Study the drawing (mm; zero at the part's minimum x, y, z) and answer. Coordinates: 2 decimals unless noted, no trailing zeros. Order: outer loops, then holes, each group sorted by start corner. A loop starts at its lowest first (then second) coordinate and runs counter-clockwise, first axis right, second up. Notation, with made-up numbers: M 35,46 L 42,46 A13 ccw 42,56 Z; hole C 42.5,76 d1. An arc over 180 degrees is marked long. Put each result on its own line as item: value.
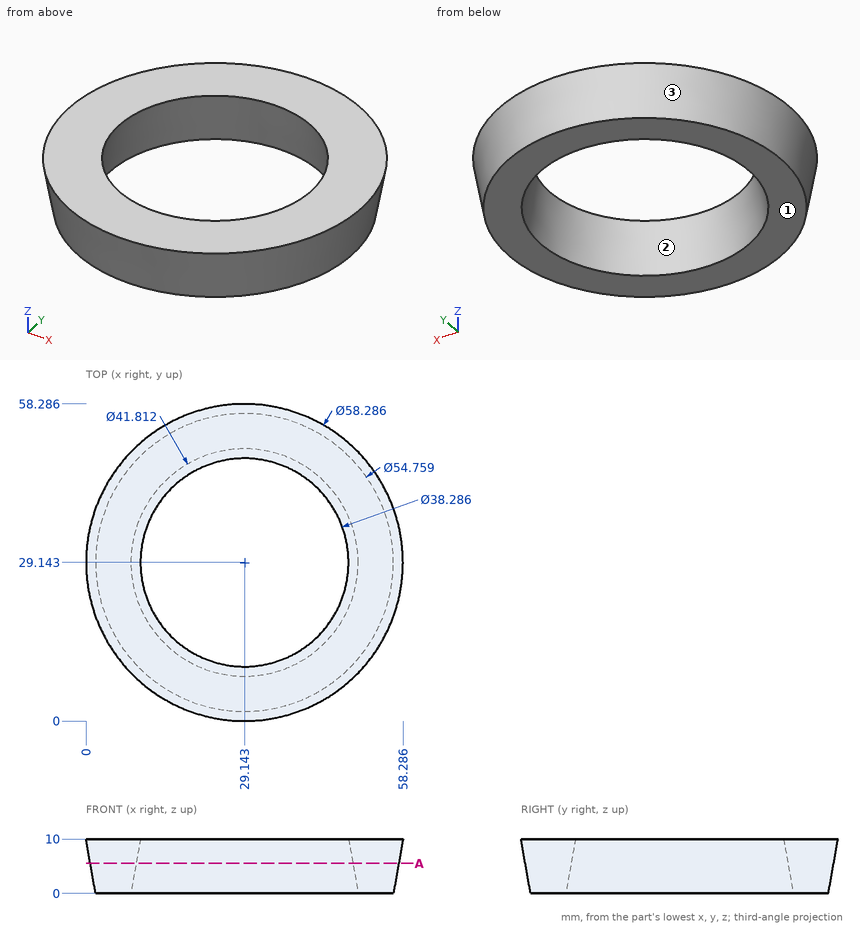
Q1. Consider line 1 along Y through (x, z) = (47.5, 6.25) (1 decimal); line 2 along Y through (x, z) = (43, 1.25) (1 decimal); line 3 along X through (y, z) = (29.5, 6.75) (1 decimal). Determine where each line is inside the solid, lowest interval first.
Answers below:
line 1: y = 7.4 to 21.7, 36.6 to 50.9
line 2: y = 5.3 to 13.8, 44.5 to 53
line 3: x = 0.6 to 9.4, 48.9 to 57.7
Q2. Given pin 1 (6 mm diameter, centred on y = 23.5, z = 6.5, fed in from -X); pin 2 (4 mm diameter, centred on x = 17.5, z = 3.5, fed in from -Y); pin 3 (1 mm diameter, centred on x = 36, z = 7.5, fed in from -Y), each flat-ended and moving along its own axis, determine where each tip first touches the part or whether it passes through.
Answers below:
pin 1: stops at x = 0.45
pin 2: stops at y = 2.77
pin 3: stops at y = 1.12
Q3. Find section A-A on z = 5.5. Write down the section's boundary in (x, y).
Answers below:
outline: C 29.14,29.14 d56.7; hole C 29.14,29.14 d39.87
Q4. For a pull along X with two mould halves and no side action, classify the marked faces 1, 2 and 3 as +X half, -X half, draft (parallel to the pull), parting line (faces both ways), or undercut.
Answers below:
face 1: draft
face 2: undercut
face 3: parting line
